The listing builds one solid part. Answer for the finished solid, in the listing's coordinates (mm). A direction names the side the tool comes from. Round coordinates to 2 decimals unless told otherwise and drop trailing zeros. Put each result on its own line as item: value. Start each with the question number.
1. Consider line 1 (Y direction, x = 0, z = -7); line 2 (Y direction, x = 0, z = -11.75); line 3 (Z direction, x = 185, y = 4.5). Determine where each line is inside the solid, lowest interval first.
2. Each of these flat-tipped pins is pushed along its axis until it touches: pin 1 Ø8 at (x, z) = (-135, -10) entering from +Y; pin 2 Ø3 at (y, z) = (-149, -10.5) entering from -X; pin 3 Ø1.5 at (y, z) = (-74, -3.5) entering from +X. Where does it stop, or does it pass through?
3. The mould has two halves that part along Y. Classify faces 4 (the face through (44.05, -198.368, -9.347)), 5 (the face through (-3, 3, 1)), 6 (the face through (26.583, 202.462, -7.471)): +Y half, -Y half, draft (parallel to the pull), parting line (faces both ways), or undercut.
4. Which of the six approach directions +Z, -Z, +X, -X, +Y, -Y give full straight-line access (tool end or side, diameter ignored) to faces 1 (the face through (45.13, -203.25, -13.37)), 2 (the face through (3, 3, 0)), 3 (the face through (137, -153, -10.846))?
from build123d import *

# Parameters (mm, degrees)
F2_R     = 67.791945
F3_DEPTH = 16.846949


with BuildPart() as f1:
    # F0 (on Front) → F1 (revolve)
    with BuildSketch(Plane.XZ):
        with BuildLine():
            Line((-199.2, 0), (0, 0))
            Line((0, 0), (0, 1))
            Line((0, 1), (-199.2, 1))
            ThreePointArc((-199.2, 1), (-202.735534, -0.464466), (-204.2, -4))
            Line((-204.2, -4), (-204.2, -10.845949))
            Line((-204.2, -10.845949), (-207.2, -10.845949))
            ThreePointArc((-207.2, -10.845949), (-207.907107, -11.138842), (-208.2, -11.845949))
            Line((-208.2, -11.845949), (-208.2, -14.845949))
            ThreePointArc((-208.2, -14.845949), (-207.907107, -15.553056), (-207.2, -15.845949))
            Line((-207.2, -15.845949), (-204.2, -15.845949))
            ThreePointArc((-204.2, -15.845949), (-203.492893, -15.553056), (-203.2, -14.845949))
            Line((-203.2, -14.845949), (-203.2, -10.845949))
            Line((-203.2, -10.845949), (-203.2, -4))
            ThreePointArc((-203.2, -4), (-202.028427, -1.171573), (-199.2, 0))
        make_face()
    revolve(axis=Axis((0, 0, 0.5), (0, 0, -1)))

    # F2 (on face) → F3 (cut, through all)
    with BuildSketch(Plane.XY.offset(1)):
        with Locations((-69.72, 70.769995)):
            Circle(F2_R)
    extrude(amount=-F3_DEPTH, mode=Mode.SUBTRACT)


solid = f1.part
Resolved:
1. line 1: -204.2 to -203.2, 203.2 to 204.2
1. line 2: -208.2 to -203.2, 203.2 to 208.2
1. line 3: 0 to 1
2. pin 1: y = 161.51
2. pin 2: x = -146.49
2. pin 3: x = 190.59
3. face 4: undercut
3. face 5: draft
3. face 6: parting line
4. face 1: +Z, -Z
4. face 2: -Z
4. face 3: +Z
